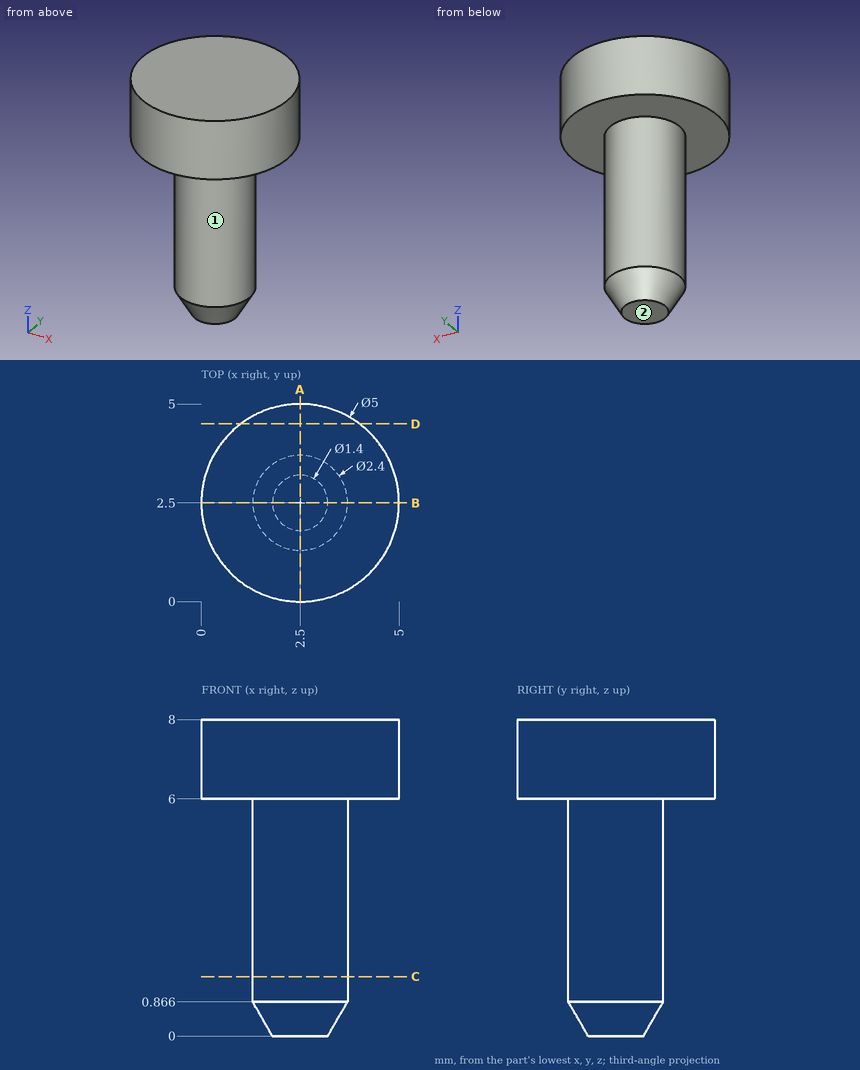
Geometry: see drawing. Coordinates: mm, zero at the bounding-box minimum. A direction names the side the tool comes from. Coordinates: 2 decimals unless noted, no trailing zeros. Loops run counter-clockwise (first coordinate to the right, second up) from the corner with the lowest first, then second, coordinate; pieces in that order, holes last. Notation, with made-up numbers: (8.5, 38) - (39.5, 38) arc R18 cw to (39.5, 70) - close; hole circle Ø3 at (-37, 8.25). An arc over 180 degrees is marked (long way). Put each result on its own line as item: value. Start each with the question number.
Q1. Cut plane A-A, the plane x = 2.5. Return loops of the section in (y, z).
Q2. Set-up query: the marked faces 1 and 2. Return all of +Z, -Z, +X, -X, +Y, -Y with unobstructed straight access to the full face (end or side cutting, diameter ignored); none if empty.
Q3. Cut plane D-D, the plane y = 4.5. Return loops of the section in (x, z), and give its area (3 significant figures).
Q4. Line query: line 1 (X direction, y = 2.55, z = 3.75); line 2 (Z direction, x = 4.2, y = 3.45); line 3 (X direction, y = 4.5, z = 6.75). Output: solid intervals per line, ascending.
Q5. Cut plane C-C, the plane z = 1.5. Return loops of the section in (x, y).
Q6. Pin query (flat end, axial travel): pin 1 Ø1.5 at (x, y) = (4.5, 1) entering from -Z; pin 2 Ø3 at (y, z) = (1, 5.5) entering from +X. Return the tip coordinate at first contact, or that it passes through.
Filled sheet:
1. outline: (0, 6) - (1.3, 6) - (1.3, 0.87) - (1.8, 0) - (3.2, 0) - (3.7, 0.87) - (3.7, 6) - (5, 6) - (5, 8) - (0, 8) - close
2. face 1: -Z
2. face 2: -Z, +X, -X, +Y, -Y
3. outline: (1, 6) - (4, 6) - (4, 8) - (1, 8) - close
3. area: 6.00 mm²
4. line 1: 1.3 to 3.7
4. line 2: 6 to 8
4. line 3: 1 to 4
5. outline: circle Ø2.4 at (2.5, 2.5)
6. pin 1: z = 6
6. pin 2: x = 5
